Check sheet for the drawn part. Datum: minimum x, y, z corner. Units: mm. Coordinates: 2 decimals unless noted, no trailing zeros. Loops run counter-clockwise (first coordinate to the right, second up) from the corner with the lowest first, then second, coordinate; pieces in that order, holes last.
Q1. Sectioned sample at B-B (x = 3). Enter the section's corners in (y, z).
Q2. Material ranges on probe 1 along X at (y, z) = (2.25, 40); probe 2 along X at (y, z) = (4.25, 15); probe 3 along Y at (x, z) = (5.5, 30), recorded low to high.
Q3. Sectioned sample at C-C (z = 19). Enter the section's corners in (x, y).
Q4. Sectioned sample at A-A (y = 2.75). Enter the section's corners in (x, z).
Q5. Go/stop test with a flat-tipped pin: P1, Ø1.5, axis at x = 2, z = 12, coming from the +Y side. Record where the tip stops, or that it passes through.
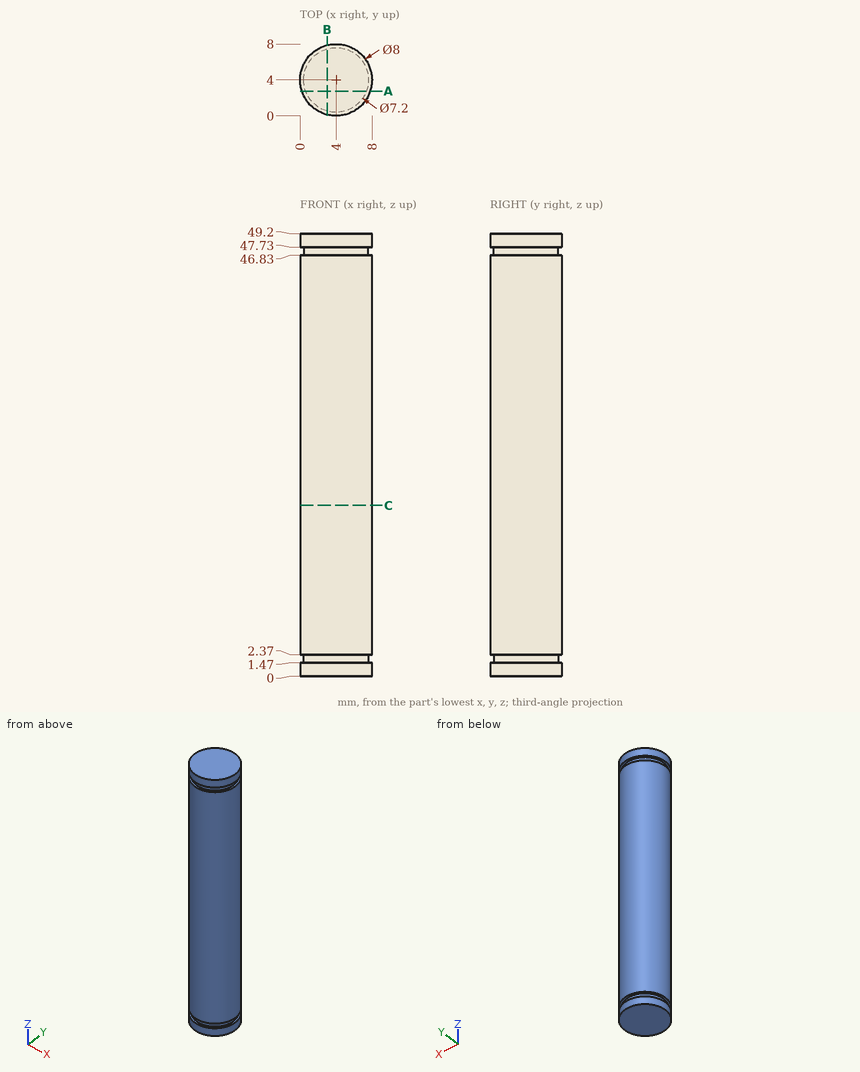
Geometry check:
1. outline: (0.13, 0) - (7.87, 0) - (7.87, 1.47) - (7.46, 1.47) - (7.46, 2.37) - (7.87, 2.37) - (7.87, 46.83) - (7.46, 46.83) - (7.46, 47.73) - (7.87, 47.73) - (7.87, 49.2) - (0.13, 49.2) - (0.13, 47.73) - (0.54, 47.73) - (0.54, 46.83) - (0.13, 46.83) - (0.13, 2.37) - (0.54, 2.37) - (0.54, 1.47) - (0.13, 1.47) - close
2. probe 1: x = 0.4 to 7.6
2. probe 2: x = 0.01 to 7.99
2. probe 3: y = 0.29 to 7.71
3. outline: circle Ø8 at (4, 4)
4. outline: (0.2, 0) - (7.8, 0) - (7.8, 1.47) - (7.38, 1.47) - (7.38, 2.37) - (7.8, 2.37) - (7.8, 46.83) - (7.38, 46.83) - (7.38, 47.73) - (7.8, 47.73) - (7.8, 49.2) - (0.2, 49.2) - (0.2, 47.73) - (0.62, 47.73) - (0.62, 46.83) - (0.2, 46.83) - (0.2, 2.37) - (0.62, 2.37) - (0.62, 1.47) - (0.2, 1.47) - close
5. P1: stops at y = 7.8
